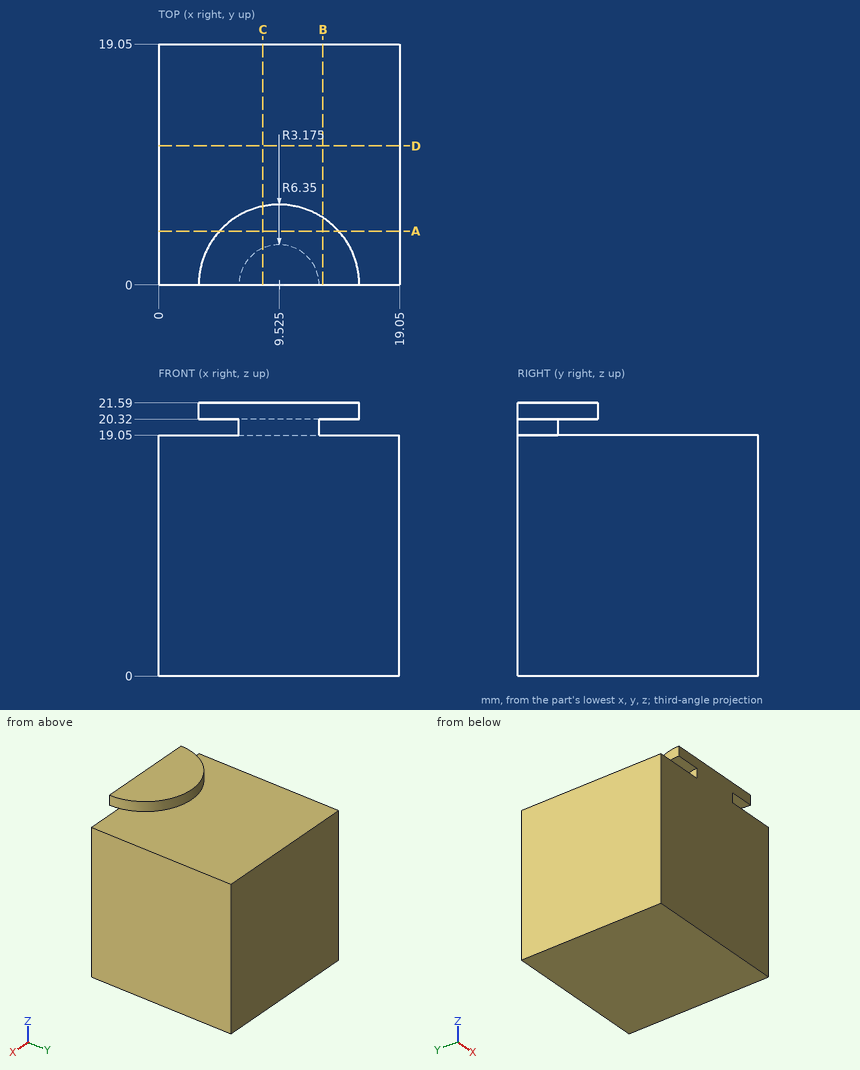
Study the drawing (mm; zero at the part's minimum x, y, z) and answer. Give positions to 0.01 mm unless a question says otherwise; leave off trailing zeros. Order: outer loops, then holes, each group sorted by start corner. A loop starts at its lowest first (then second) coordinate and runs counter-clockwise, first axis right, second up.
1. Section C-C, the plane x = 8.25 is taken. Determine the outline of the cut face in (y, z), and give its area (3 significant figures).
Result sheet:
outline: (0, 0) - (19.05, 0) - (19.05, 19.05) - (2.91, 19.05) - (2.91, 20.32) - (6.22, 20.32) - (6.22, 21.59) - (0, 21.59) - close
area: 374 mm2
2. Section B-B, the plane x = 13 is taken. Determine the outline of the cut face in (y, z), and give its area (3 significant figures).
Result sheet:
outline: (0, 0) - (19.05, 0) - (19.05, 19.05) - (0, 19.05) - close; (0, 20.32) - (5.31, 20.32) - (5.31, 21.59) - (0, 21.59) - close
area: 370 mm2
3. Section D-D, the plane y = 11 is taken. Determine the outline of the cut face in (x, z), and give its area (3 significant figures).
Result sheet:
outline: (0, 0) - (19.05, 0) - (19.05, 19.05) - (0, 19.05) - close
area: 363 mm2
4. Straight lines are drawn through the part: L1, parallel to Z at x = 9.75, y = 7.5; L2, parallel to Y at x = 9.25, z = 20. For each, find the intervals that lie inside material, in ascending order.
Result sheet:
L1: z = 0 to 19.05
L2: y = 0 to 3.16
5. Section A-A, the plane y = 4.25 is taken. Determine the outline of the cut face in (x, z).
Result sheet:
outline: (0, 0) - (19.05, 0) - (19.05, 19.05) - (0, 19.05) - close; (4.81, 20.32) - (14.24, 20.32) - (14.24, 21.59) - (4.81, 21.59) - close
6. This flat-tipped pin is pushed along its axis until it touches: P1, Ø1.5, axis at x = 12, y = 13, coming from the +Z side. Where does it stop, or does it pass through?
Result sheet:
P1: stops at z = 19.05
